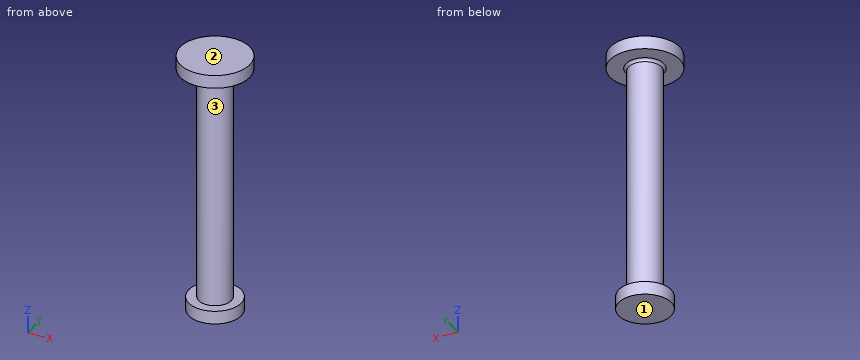
Autodesk Inventor part; units mm, degrees
ref_plane "YZ Plane" through (0, 0, 0) normal (1, 0, 0) x (0, 1, 0)
ref_plane "XZ Plane" through (0, 0, 0) normal (0, 1, 0) x (-1, 0, 0)
ref_plane "XY Plane" through (0, 0, 0) normal (0, 0, 1) x (1, 0, 0)
sketch "Sketch1" plane through (0, 0, 0) normal (0, 0, 1) x (1, 0, 0)
  circle A0 centre (0, 0) radius 12.5
  dimension "d0" = 25
extrude "Extrusion1" add sketch "Sketch1" along normal blind 180
sketch "Sketch2" plane through (0, 0, 180) normal (0, 0, 1) x (1, 0, 0)
  circle A0 centre (0, 0) radius 26.5
  dimension "d3" = 53
extrude "Extrusion2" add sketch "Sketch2" along normal blind 10
fillet "Fillet1" radius 2 1 edges at (-12.5, 0, 180)
sketch "Sketch3" plane through (0, 0, 0) normal (0, 0, -1) x (-1, 0, 0)
  circle A0 centre (0, 0) radius 20
  dimension "d7" = 40
extrude "Extrusion3" add sketch "Sketch3" along normal blind 10
properties part number "PISTON"
Check sheet for the modelled part. Datum: model origin and axes. Units: mm. Face numbers are marked on the shaded views. Round coordinates to 2 decimals unless told otherwise and drop trailing zeros. Order: outer loops, then holes, each group sorted by start corner. A loop starts at its lowest first (then second) coordinate and runs counter-clockwise, first axis right, second up. Notation, with made-up numbers: (-13.5, -11.5) -> (20.5, -11.5) arc R32 cw to (20.5, 22.5) -> close; hole circle Ø2 at (64.25, 8.5). An arc over 180 degrees is marked (long way). One line per item, written item: value. Start each with the question number.
Q1. Cross-section at D-D (z = 19). Record the boundary of the cut face in (x, y), and give its area (3 significant figures).
Q2. Gauge pin test, flat ends, axial feed: pin 1 Ø12 at (y, z) = (-16.5, 150.5) entering from +X; pin 2 Ø4 at (x, z) = (13, 11) entering from -Y; pin 3 Ø3 at (y, z) = (-11.5, 130) entering from -X. Record the tip position at first contact, or that the pin passes through.
Q3. Mould release check, pull along Z, two halves, no side actions. Record for the marked faces 1, 2 and 3: pulls with the +Z half, pulls with the -Z half, needs draft (parallel to the pull), parting line crosses it, or undercut.
Q4. Cross-section at A-A (x = 16.5). Record the boundary of the cut face in (y, z).
Q5. Thickness scan on line 1 (Z direction, x = -17.5, y = 1); line 2 (Z direction, x = -15, y = -16); line 3 (Y direction, x = 0, z = 163.5). Record the ranges inside material, lowest first.
Q6. Cross-section at B-B (y = 0). Record the boundary of the cut face in (x, z).
Completed:
1. outline: circle Ø25 at (0, 0)
1. area: 491 mm²
2. pin 1: stops at x = 6.78
2. pin 2: stops at y = -5.94
2. pin 3: stops at x = -7.5
3. face 1: pulls with the -Z half
3. face 2: pulls with the +Z half
3. face 3: undercut
4. outline: (-20.74, 180) -> (20.74, 180) -> (20.74, 190) -> (-20.74, 190) -> close; (-11.3, -10) -> (11.3, -10) -> (11.3, 0) -> (-11.3, 0) -> close
5. line 1: z = -10 to 0, 180 to 190
5. line 2: z = 180 to 190
5. line 3: y = -12.5 to 12.5
6. outline: (-26.5, 180) -> (-14.5, 180) arc R2 cw to (-12.5, 178) -> (-12.5, 0) -> (-20, 0) -> (-20, -10) -> (20, -10) -> (20, 0) -> (12.5, 0) -> (12.5, 178) arc R2 cw to (14.5, 180) -> (26.5, 180) -> (26.5, 190) -> (-26.5, 190) -> close
